from build123d import *

# Parameters (mm, degrees)
F1_DEPTH = 18
F2_W     = 18
F2_H     = 4
F3_DEPTH = 20


with BuildPart() as f1:
    # F0 (on Front) → F1 (new body)
    with BuildSketch(Plane.XZ):
        Polygon((55, 96.89723), (0, 96.89723), (-55, 96.89723), (-53.852537, 103.404814), (-66.037657, 103.404814), (-84.270715, 0), (-72.085596, 0), (-56.410616, 88.89723), (0, 88.89723), (56.410616, 88.89723), (72.085596, 0), (84.270715, 0), (66.037657, 103.404814), (53.852537, 103.404814), align=None)
    extrude(amount=F1_DEPTH)

    # F2 (on face) → F3 (cut)
    with BuildSketch(Plane.XZ.offset(18)):
        with Locations((0, 90.89723)):
            Rectangle(F2_W, F2_H)
    extrude(amount=-F3_DEPTH, mode=Mode.SUBTRACT)


solid = f1.part
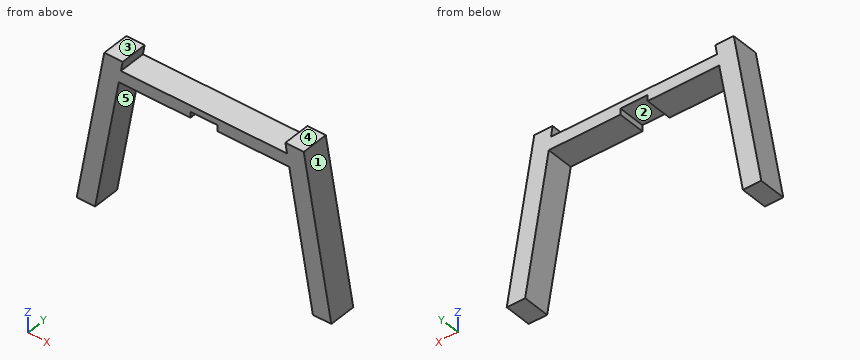
Model file for the job. Use its own axes, mm. Face numbers are marked on the shaded views. A direction names the side the tool comes from. Give positions to 0.01 mm unless a question says otherwise; leave off trailing zeros. Order: outer loops, then holes, each group sorted by start corner. A loop starts at its lowest first (then second) coordinate and runs counter-clockwise, first axis right, second up. Notation, with made-up numbers: M 78.5,-9.5 L 121.5,-9.5 A26 ccw 121.5,10.5 Z; hole C 32,7.25 d7. An arc over 180 degrees is marked long. Put each result on its own line as item: value. Start each with the question number.
(1) Band-saw the part on A-A on z = 82. Give the cut face in (x, y).
(2) Band-saw the part on D-D on x = -60.5. Give the cut face in (y, z).
(3) Band-saw the part on B-B on y = -1.75. Give the cut face in (x, z).
(4) Tool access for the marked faces 4 and 5: list every direction of +Z, -Z, +X, -X, +Y, -Y with a clear straight run to the whole face (end or side of a thin tool).
(5) Pull direction X, two halves, no side cores. Call the marked faces 1, 2 and 3: released by +X, released by -X, zero draft, split by the parting line, or undercut.
(6) Drill centre lines: L1, parallel to Z at x = 44.5, y = -11.75; L2, parallel to X at y = -9.25, z = 27.5; L3, parallel to Z at x = 8.5, y = -6.75. Where is each one in solid material? Low to high. Write a range as [from, to].
(7) Pin check, flat tips, straight feed: pin 1 Ø1.2 at (y, z) = (-11, 91.5) entering from +X; pin 2 Ø10 at (x, y) = (-18, -11.5) entering from -Z; pin 3 Ø6 at (y, z) = (-11, 51) entering from -X. Stop position of each tip, or through.
(8) Band-saw the part on C-C on x = -36. Give the cut face in (y, z).
Results below:
1. outline: M -69.81,-18 L -57.63,-18 L -57.63,0 L -69.81,0 Z; M 57.63,-18 L 69.81,-18 L 69.81,0 L 57.63,0 Z
2. outline: M -18,65.71 L 0,65.71 L 0,103.4 L -18,103.4 Z
3. outline: M -84.27,0 L -72.09,0 L -56.41,88.9 L -9,88.9 L -9,92.9 L 9,92.9 L 9,88.9 L 56.41,88.9 L 72.09,0 L 84.27,0 L 66.04,103.4 L 53.85,103.4 L 55,96.9 L -55,96.9 L -53.85,103.4 L -66.04,103.4 Z
4. face 4: +Z, +X, -X, +Y, -Y
4. face 5: -Z, +Y, -Y
5. face 1: released by +X
5. face 2: undercut
5. face 3: zero draft
6. L1: z = [88.9, 96.9]
6. L2: x = [-79.42, -67.24], [67.24, 79.42]
6. L3: z = [92.9, 96.9]
7. pin 1: stops at x = 68.24
7. pin 2: stops at z = 88.9
7. pin 3: stops at x = -75.81
8. outline: M -18,88.9 L 0,88.9 L 0,96.9 L -18,96.9 Z
